Autodesk Inventor part; units mm, degrees
ref_plane "РабПлоскость1" through (8.55, 0, 0) normal (1, 0, 0) x (0, 0, -1)
ref_plane "YZ Plane" through (0, 0, 0) normal (1, 0, 0) x (0, 1, 0)
ref_plane "XZ Plane" through (0, 0, 0) normal (0, 1, 0) x (-1, 0, 0)
sketch "Эскиз1" plane through (0, 0, 0) normal (0, 1, 0) x (-1, 0, 0)
  line L0 (0, 0) -> (-17.1, 0)
  line L1 (-17.1, 0) -> (-17.1, -35.8)
  line L2 (-17.1, -35.8) -> (0, -35.8)
  line L3 (0, -35.8) -> (0, 0)
  dimension "d0" = 17.1
  dimension "d1" = 35.8
extrude "Выдавливание1" add sketch "Эскиз1" along normal blind 0.75
sketch "Эскиз2" plane through (0, 0.75, 0) normal (0, 1, 0) x (1, 0, 0)
  line L0 (0, 35.8) -> (0, 0)
  line L1 (17.1, 0) -> (17.1, 35.8)
  line L2 (0, 35.8) -> (17.1, 35.8)
  line L3 (17.1, 35.8) -> (17.1, 3.2)
  line L4 (17.1, 3.2) -> (0, 3.2)
  line L5 (0, 3.2) -> (0, 35.8)
  point P0 (0, 3.2)
  dimension "d4" = 32.6
extrude "Выдавливание2" add sketch "Эскиз2" along normal blind 0.75
sketch "Эскиз3" plane through (0, 0, 0) normal (0, -1, 0) x (1, 0, 0)
  line L0 (0, -35.8) -> (0, -3.2)
  line L1 (0, -3.2) -> (17.1, -3.2)
  line L2 (17.1, -3.2) -> (17.1, -35.8)
  line L3 (17.1, -35.8) -> (0, -35.8)
  line L4 (15.9, -34.2) -> (1.2, -34.2)
  line L5 (1.2, -34.2) -> (1.2, -4.8)
  line L6 (1.2, -4.8) -> (15.9, -4.8)
  line L7 (15.9, -4.8) -> (15.9, -34.2)
  point P0 (0, 0)
  point P1 (8.55, -34.2)
  point P2 (8.55, -35.8)
  point P3 (15.9, -19.5)
  point P4 (17.1, -19.5)
  dimension "d7" = 29.4
  dimension "d8" = 14.7
extrude "Выдавливание3" cut sketch "Эскиз3" against normal blind 0.01 contours L4 L5 L6 L7
ref_plane "РабПлоскость1" through (8.55, 0, 0) normal (1, 0, 0) x (0, 0, -1)
sketch "Эскиз4" plane through (8.55, 0, 0) normal (1, 0, 0) x (0, 0, -1)
  line L0 (0, 0) -> (0, 0.75)
  arc A0 (0, 4.75) -> (0, 0.75) centre (0, 2.75) ccw
  arc A1 (0, 4.85) -> (0, 0.65) centre (0, 2.75) ccw
  line L1 (0, 4.75) -> (5.0168, 4.75)
  line L2 (5.0168, 4.75) -> (5.0168, 4.85)
  line L3 (5.0168, 4.85) -> (0, 4.85)
  dimension "d11" = 0.1
  dimension "d12" = 2
  dimension "d13" = 5.0168
extrude "Выдавливание4" add sketch "Эскиз4" along normal mid plane 9.3
properties part number "Display_1.3"
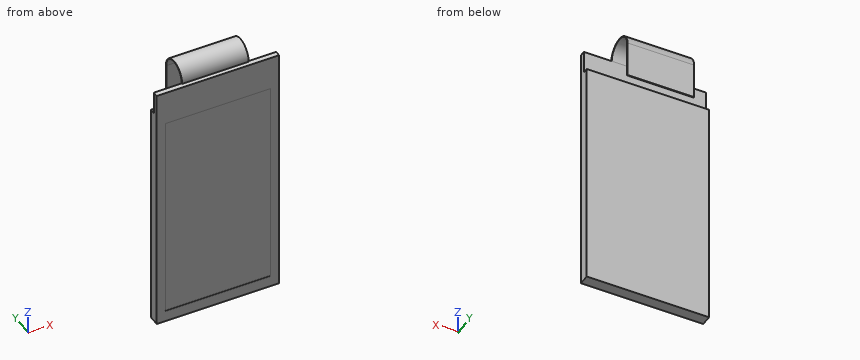
Verification items for the finished model (mm, model axes). Give positions to 0.01 mm unless a question says otherwise; leave off trailing zeros. Loops run counter-clockwise (first coordinate to the right, second up) from the corner with the lowest first, then second, coordinate; pieces in that order, holes last.
1) Sectioned sample at D-D, the plane y = 2.75. Enter the section's corners in (x, z).
2) Depth check by flat-ended pin: pin 1 Ø5.5 at (x, z) = (7.5, -1.5) entering from -Y; pin 2 Ø0.8 at (x, y) = (6.5, 1) entering from +Z; pin 3 Ø1.5 at (y, z) = (2.5, -28) entering from -X; pin 4 Ø0.8 at (x, y) = (12, 0.5) entering from +Z. Enter the tip coordinate at first touch or a pass-through.
3) Thickness scan on line 1 along Y through (x, z) = (8.25, -15.5); line 2 along Z through (x, y) = (10.75, 0.35); line 3 along Z through (x, y) = (5.75, 4.5). Record the ranges inside material, lowest first.
Answers:
1. outline: (3.9, 2) - (13.2, 2) - (13.2, 2.1) - (3.9, 2.1) - close
2. pin 1: stops at y = 0
2. pin 2: stops at z = 1.61
2. pin 3: passes through
2. pin 4: stops at z = 0.99
3. line 1: y = 0.01 to 1.5
3. line 2: z = -35.8 to 0
3. line 3: z = 0.97 to 1.16
